```python
from build123d import *

# Parameters (mm, degrees)
F1_DEPTH      = 19.05
F3_D          = 6.35
F5_DEPTH      = 6.35
F5_DEPTH_BACK = 10.2098643316
F6_W          = 4.7625
F6_H          = 5.08
F7_DEPTH      = 25.4
F8_R          = 1.5875
F9_DEPTH      = 6.35
F11_START     = 3.175
F11_DEPTH     = 15.875
F13_DEPTH     = 19.0510001


with BuildPart() as f1:
    # F0 (on Right) → F1 (new body)
    with BuildSketch(Plane.YZ):
        with BuildLine():
            ThreePointArc((-3.9967504682, -1.0709260603), (-1.8851834207, 0.7808685404), (-2.0688702794, 3.5833884382))
            Line((-2.0688702794, 3.5833884382), (-36.2669128953, 62.8161357684))
            ThreePointArc((-36.2669128953, 62.8161357684), (-38.5911742094, 65.1403970824), (-41.7661742094, 65.9911357684))
            Line((-41.7661742094, 65.9911357684), (-47.625, 65.9911357684))
            Line((-47.625, 65.9911357684), (-47.625, -10.2088642316))
            Line((-47.625, -10.2088642316), (-38.9359933597, -10.2088642316))
            ThreePointArc((-38.9359933597, -10.2088642316), (-38.1071520391, -10.1545391013), (-37.2924924233, -9.9924932286))
            Line((-37.2924924233, -9.9924932286), (-3.9967504682, -1.0709260603))
        make_face()
    extrude(amount=F1_DEPTH)

    # F3 (through all)
    with Locations(Plane(origin=(0, 0, -10.2088642316), x_dir=(1, 0, 0), z_dir=(0, 0, -1))):
        with Locations((9.525, 42.8625)):
            Hole(F3_D / 2)

    # F4 (on Top) → F5 (cut, two sides)
    with BuildSketch(Plane.XY) as f5_sk:
        with BuildLine():
            Line((15.8740343467, -1.5875), (0, -1.5875))
            ThreePointArc((0, -1.5875), (-11.1632427706, -28.7495561195), (15.8740343467, -17.2874041455))
            Line((15.8740343467, -17.2874041455), (15.8740343467, -10.9579507262))
            Line((15.8740343467, -10.9579507262), (15.8740343467, -1.5875))
        make_face()
    extrude(amount=F5_DEPTH, mode=Mode.SUBTRACT)
    extrude(f5_sk.sketch, amount=-F5_DEPTH_BACK, mode=Mode.SUBTRACT)

    # F6 (on face) → F7 (cut)
    with BuildSketch(Plane(origin=(15.8740343467, 0, 0), x_dir=(0, -1, 0), z_dir=(-1, 0, 0))):
        with Locations((14.9061541455, 1.42875)):
            Rectangle(F6_W, F6_H)
    extrude(amount=-F7_DEPTH, mode=Mode.SUBTRACT)

    # F8 (on face) → F9 (cut)
    with BuildSketch(Plane(origin=(0, 0, 0), x_dir=(0, -1, 0), z_dir=(-1, 0, 0))):
        with Locations((36.5125, 3.96875)):
            Circle(F8_R)
    extrude(amount=-F9_DEPTH, mode=Mode.SUBTRACT)

    # F10 (on face) → F11 (join)
    with BuildSketch(Plane(origin=(0, 0, 6.35), x_dir=(1, 0, 0), z_dir=(0, 0, -1)).offset(F11_START)):
        with BuildLine():
            ThreePointArc((1.5875, 25.2249041455), (3.4473719395, 20.7347760849), (7.9375, 18.8749041455))
            Line((7.9375, 18.8749041455), (15.8120441288, 18.8749041455))
            ThreePointArc((15.8120441288, 18.8749041455), (11.2873318483, 28.6254639767), (1.5875, 33.2579255641))
            Line((1.5875, 33.2579255641), (1.5875, 25.2249041455))
        make_face()
    extrude(amount=F11_DEPTH)

    # F12 (on face) → F13 (cut, through all)
    with BuildSketch(Plane.YZ.offset(19.05)):
        Polygon((-14.8947556834, -3.9910377568), (-34.9698544916, -9.3701442705), (-35.4003421962, -17.2549132258), (-14.8947556834, -17.2549132258), align=None)
    extrude(amount=-F13_DEPTH, mode=Mode.SUBTRACT)


solid = f1.part
```
Geometry check sheet. Reference: the model listing, model coordinates, mm. A direction names the side the tool comes from. Give positions to 0.01 mm unless a question says otherwise; leave off trailing zeros. Order: outer loops, then holes, each group sorted by start corner. A loop starts at its lowest first (then second) coordinate and runs counter-clockwise, first axis right, second up. Notation, with made-up numbers: (-24, 10) - (-16, 10) arc R38 ccw to (-16, 49) - close; hole circle Ø1 at (16, 16). An arc over 180 degrees is marked (long way). Write item = value, one per line. Start each with the question number.
1) Access from +Z, -Z, +X, -X, +Y, -Y to the whole of each face (thin tool, end or side, straight path). Record for faces 1 (the cylindrical face through (3.131, -35.253, 3.003)), 2 (the flat face through (12, -18.875, -1)), 3 (the flat face through (17, -15, 3.969)), 4 (the cylindrical face through (9.392, -38.119, -10.156)), 5 (the flat face through (7, -25, 3.175)).
2) Scan lines: L1, parallel to X at y = -43, z = 37.5; L2, parallel to X at y = -11, z = 5; L3, parallel to Y at x = 7.75, z = 4 (3 decimals). Record each from-to range of solid material in increasing order.
3) Section check C-C (y = -40.5). Enter the section's corners in (x, z), then the cut area to 3 significant figures.
4) Section check D-D (y = -21). Enter the section's corners in (x, z) (3 decimals).
5) Draft check along X on faces 6 (the flat face through (15.874, -10, 2)), 7 (the cylindrical face through (10, -46, 28)), 8 (the cylindrical face through (17.44, -1.901, 0.743)). Enter one of: released by +X, released by -X, zero draft, split by the parting line, or undercut.
6) Gauge pin test, flat ends, axial feed: pin 1 Ø1.6 at (y, z) = (-37, 4.5) entering from -X; pin 2 Ø7 at (x, y) = (9, -29) entering from +Z; pin 3 Ø3 at (x, z) = (12.5, 42) entering from +Y. Record the tip position at first contact, or that the pin passes through.
Geometry check:
q1.face_1 = -X
q1.face_2 = -Z, -X, +Y
q1.face_3 = +X, -X
q1.face_4 = -Z, +X, -X, +Y
q1.face_5 = -X, +Y
q2.L1 = 0 to 6.35, 12.7 to 19.05
q2.L2 = 15.87 to 19.05
q2.L3 = -47.625 to -45.495, -40.23 to -31.317
q3.outline = (0, -10.21) - (7.4, -10.21) - (7.4, 65.86) - (0, 65.86) - close; (11.65, -10.21) - (19.05, -10.21) - (19.05, 65.86) - (11.65, 65.86) - close
q3.area = 1,130 mm2
q4.outline = (0, 6.35) - (15.476, 6.35) - (15.476, 3.175) - (3.197, 3.175) - (3.197, -5.627) - (19.05, -5.627) - (19.05, 36.373) - (0, 36.373) - close
q5.face_6 = released by -X
q5.face_7 = undercut
q5.face_8 = zero draft
q6.pin_1 = 6.35
q6.pin_2 = 56.29
q6.pin_3 = -23.38
